Check sheet for the modelled part. Datum: model origin and axes. Units: mm. A direction names the side the tool comes from. Give positions to 0.01 mm unless a question says otherwise; leave off trailing zeros. Loops run counter-clockwise (first coordinate to the right, second up) from the corner with the lowest first, then second, coordinate; pieces in that order, holes last. Notation, with made-up numbers: (-29, 68.25) -> (16, 68.25) arc R26 ccw to (16, 92.25) -> close; hole circle Ø3 at (68.5, 46). An arc over 180 degrees is marked (long way). Answer as CSV lines item,"result". Start each with the question number.
(1) Section check C-C on y = -8. Enter the section's corners in (x, z).
(2) Gauge pin test, flat ends, axial feed: pin 1 Ø3 at (x, z) = (-1, -14.5) entering from +Y; pin 2 Ø1 at (x, z) = (-0.5, 7.5) entering from -Y; pin 3 Ø24 at (y, z) = (0, 0) entering from +X. Record the tip position at first contact, or that the pin passes through.
(3) Material ranges on line 1 (Y direction, x = -3.75, z = 0); line 2 (Y direction, x = -4.75, z = 19); line 3 (Z direction, x = -5.75, y = 3.5), recorded low to high. Write a range as from..to.
(4) Access from +Z, -Z, +X, -X, +Y, -Y to the whole of each face (thin tool, end or side, straight path). Record for faces 1 (the face through (-2.38, 21.924, 19.771)), 2 (the face through (0.08, -0.88, -19.98)).
(5) Section check D-D on x = 1.25. State how many separate pieces and enclosed holes the cut face has, plus the area to 3 significant figures.
(6) Section check A-A on y = 0. Enter the section's corners in (x, z).
(7) Release check for a two-part mould opening along Y. For faces 3 (the face through (-2, 0, 30)), 4 (the face through (-7.45, 8, 8)), 5 (the face through (-2.52, -1.76, -39.96)) record: pulls with the +Y half, pulls with the -Y half, needs draft (parallel to the pull), parting line crosses it, or undercut.
(8) Section check B-B on z = -27.5. Enter the section's corners in (x, y).
from build123d import *

# Parameters (mm, degrees)
SKETCH2_R          = 2.5
CUT_EXTRUDE1_DEPTH = 58.445626465


with BuildPart() as part:
    # Sketch1 → Revolve1 (revolve)
    with BuildSketch(Plane.XY, mode=Mode.PRIVATE) as revolve1_sk:
        Polygon((2.55, 20), (2.55, 40), (-7.45, 40), (-7.45, 11), (-2.45, 11), (-2.45, 20), align=None)
    revolve(revolve1_sk.sketch.rotate(Axis((-7.45, 0, 0), (1, 0, 0)), 90), axis=Axis((-7.45, 0, 0), (1, 0, 0)))

    # Sketch2 → Cut-Extrude1 (cut, through all)
    with BuildSketch(Plane(origin=(2.55, 0, 0), x_dir=(0, 0, -1), z_dir=(1, 0, 0))):
        with Locations((-19.445436483, -19.445436483)):
            Circle(SKETCH2_R)
        with Locations((-27.5, 0)):
            Circle(SKETCH2_R)
        with Locations((-19.445436483, 19.445436483)):
            Circle(SKETCH2_R)
        with Locations((0, 27.5)):
            Circle(SKETCH2_R)
        with Locations((19.445436483, 19.445436483)):
            Circle(SKETCH2_R)
        with Locations((27.5, 0)):
            Circle(SKETCH2_R)
        with Locations((19.445436483, -19.445436483)):
            Circle(SKETCH2_R)
        with Locations((0, -27.5)):
            Circle(SKETCH2_R)
    extrude(amount=-CUT_EXTRUDE1_DEPTH, mode=Mode.SUBTRACT)


solid = part.part
Working result:
1,outline,"(-7.45, -39.19) -> (2.55, -39.19) -> (2.55, -18.33) -> (-2.45, -18.33) -> (-2.45, -7.55) -> (-7.45, -7.55) -> close; (-7.45, 7.55) -> (-2.45, 7.55) -> (-2.45, 18.33) -> (2.55, 18.33) -> (2.55, 39.19) -> (-7.45, 39.19) -> close"
2,pin 1,"stops at y = 37.83"
2,pin 2,"stops at y = -39.38"
2,pin 3,"stops at x = -2.45"
3,line 1,"y = -40..-30, -25..-11, 11..25, 30..40"
3,line 2,"y = -35.2..-21.91, -16.99..16.99, 21.91..35.2"
3,line 3,"z = -39.85..-10.43, 10.43..39.85"
4,face 1,"+X, -X"
4,face 2,"+X"
5,separate pieces,"1"
5,enclosed holes,"9"
5,area,"3,610 mm^2"
6,outline,"(-7.45, -40) -> (2.55, -40) -> (2.55, -30) -> (-7.45, -30) -> close; (-7.45, -25) -> (2.55, -25) -> (2.55, -20) -> (-2.45, -20) -> (-2.45, -11) -> (-7.45, -11) -> close; (-7.45, 11) -> (-2.45, 11) -> (-2.45, 20) -> (2.55, 20) -> (2.55, 25) -> (-7.45, 25) -> close; (-7.45, 30) -> (2.55, 30) -> (2.55, 40) -> (-7.45, 40) -> close"
7,face 3,"undercut"
7,face 4,"needs draft"
7,face 5,"parting line crosses it"
8,outline,"(-7.45, -29.05) -> (2.55, -29.05) -> (2.55, -2.5) -> (-7.45, -2.5) -> close; (-7.45, 2.5) -> (2.55, 2.5) -> (2.55, 29.05) -> (-7.45, 29.05) -> close"
